Design review of the part shown in the three views and the two pictorial views. Dimensions are in mm from the part's minimum x, y and z. A direction names the side the tool comes from. Coordinates: 2 decimals unless noted, no trailing zeros. Loops run counter-clockwise (first coordinate to the right, second up) from the corner with the lowest first, then second, coordinate; pieces in that order, holes last. Notation, with made-up numbers: (62, 49) -> (100, 49) arc R18 ccw to (100, 58) -> close; hole circle Ø9 at (1.5, 1.5). An arc over 180 degrees is marked (long way). Answer in a Markdown table with one row per item.
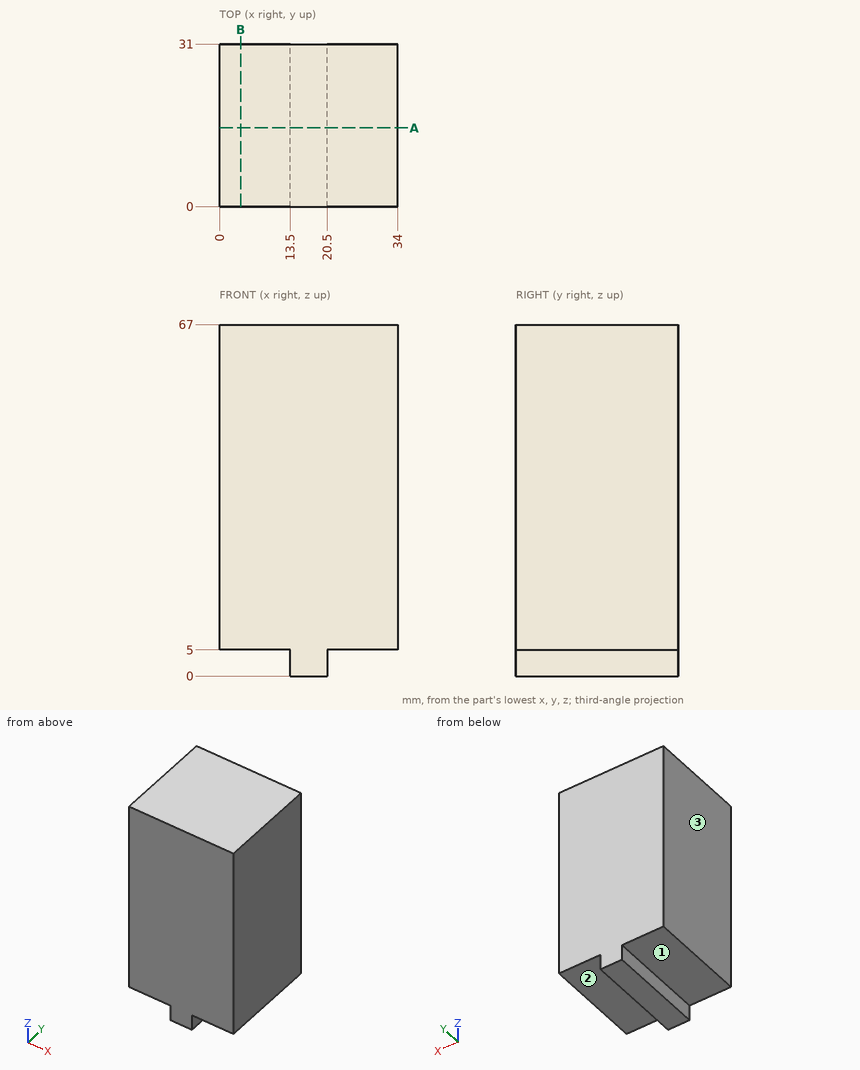
Item 1: Take a section at B-B, the plane x = 4. State the section outline as (y, z) points, and give its area (3 significant figures).
Worked answers:
| item | result |
|---|---|
| outline | (0, 5) -> (31, 5) -> (31, 67) -> (0, 67) -> close |
| area | 1,920 mm² |
Item 2: Take a section at A-A, the plane y = 15. State the section outline as (x, z) points.
Worked answers:
| item | result |
|---|---|
| outline | (0, 5) -> (13.5, 5) -> (13.5, 0) -> (20.5, 0) -> (20.5, 5) -> (34, 5) -> (34, 67) -> (0, 67) -> close |
Item 3: Insertion check: pin 1 (7 mm diameter, centred on x = 8.5, y = 8.5, fed in from -Z); pin 2 (1.5 mm diameter, centred on y = 10, z = 2, fed in from +X); pin 3 (1.5 mm diameter, centred on y = 19, z = 3.5, fed in from -X). Each pin has a flat end and moves straight along its axis. Give the tip position at first contact, or say it passes through.
Worked answers:
| item | result |
|---|---|
| pin 1 | z = 5 |
| pin 2 | x = 20.5 |
| pin 3 | x = 13.5 |
Item 4: For L1, parallel to Z at x = 22.5, y = 26, list the stretches that pass through material, from the lowest coordinate up.
Worked answers:
| item | result |
|---|---|
| L1 | 5 to 67 |
Item 5: For the marked faces 1, 2 and 3, list the 3-axis set-ups (+Z, -Z, +X, -X, +Y, -Y) from which the entire face can be reached by the end or side of a thin tool; tool diameter is ignored.
Worked answers:
| item | result |
|---|---|
| face 1 | -Z, -X, +Y, -Y |
| face 2 | -Z, +X, +Y, -Y |
| face 3 | +Z, -Z, -X, +Y, -Y |
